from build123d import *

# Parameters (mm, degrees)
SKETCH1_W                = 50
SKETCH1_H                = 100
BOSS_EXTRUDE1_DEPTH      = 2.5
BOSS_EXTRUDE1_DEPTH_BACK = 2.5


with BuildPart() as part:
    # Sketch1 → Boss-Extrude1 (new body, two sides)
    with BuildSketch(Plane(origin=(0, 0, 0), x_dir=(1, 0, 0), z_dir=(0, 1, 0))) as boss_extrude1_sk:
        Rectangle(SKETCH1_W, SKETCH1_H)
        with BuildLine():
            Line((4.7625, 35.2375), (4.7625, -35.2375))
            ThreePointArc((4.7625, -35.2375), (0, -40), (-4.7625, -35.2375))
            Line((-4.7625, -35.2375), (-4.7625, 35.2375))
            ThreePointArc((-4.7625, 35.2375), (0, 40), (4.7625, 35.2375))
        make_face(mode=Mode.SUBTRACT)
    extrude(amount=BOSS_EXTRUDE1_DEPTH)
    extrude(boss_extrude1_sk.sketch, amount=-BOSS_EXTRUDE1_DEPTH_BACK)


solid = part.part
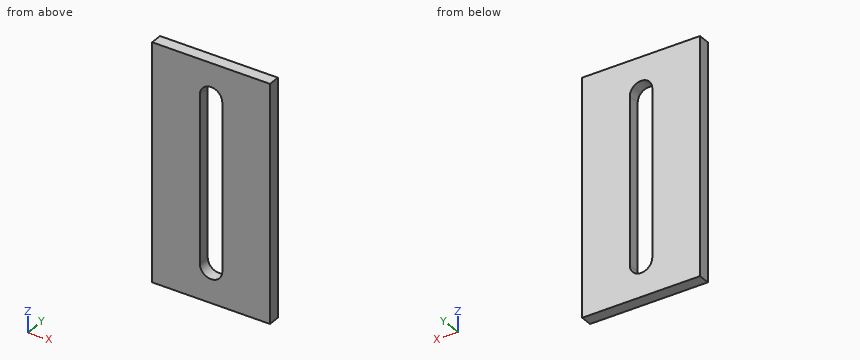
The listing builds one solid part. Answer for the finished solid, in the listing's coordinates (mm). Round coordinates to 2 decimals unless told otherwise and drop trailing zeros. Write each loop counter-clockwise with the first axis right and the second up, starting at its lowest first coordinate (ties: lowest second). Pieces come first, ordered by that corner, then holes. Notation, with made-up numbers: M -24,0 L 5,0 A14 ccw 5,27 Z; hole C -34.75,35.25 d3. An arc over 180 degrees is marked long. Write each question's results on one line, items separated by ' | '. Start each with the question number.
(1) The part is cut by section C-C, the plane z = 12.5. Write down the section's boundary in (x, y), and give its area (3 significant figures).
(2) Each of these flat-tipped pins is pushed along its axis until it touches: P1, Ø12, axis at x = 3.5, z = -4.5, coming from the +Y side; P2, Ø1, axis at x = 4, z = 36, coming from the -Y side. Where does it stop, or does it pass through?
(3) The part is cut by section A-A, the plane x = 0. Write down the section's boundary in (y, z).
(4) The part is cut by section B-B, the plane y = -1.35. Write down the section's boundary in (x, z) (1 decimal), and give its area (3 significant figures).
(5) Find the intervals of material crossed by line 1 (X direction, y = 1.9, z = 23); line 2 (X direction, y = -0.3, z = -37); line 3 (Z direction, x = 4, y = -0.5), in increasing order.
Worked answers:
1) outline: M -25,-2.5 L -4.76,-2.5 L -4.76,2.5 L -25,2.5 Z; M 4.76,-2.5 L 25,-2.5 L 25,2.5 L 4.76,2.5 Z | area: 202 mm²
2) P1: stops at y = 2.5 | P2: passes through
3) outline: M -2.5,-50 L 2.5,-50 L 2.5,-40 L -2.5,-40 Z; M -2.5,40 L 2.5,40 L 2.5,50 L -2.5,50 Z
4) outline: M -25,-50 L 25,-50 L 25,50 L -25,50 Z; hole M -4.8,-35.2 A4.8 ccw 4.8,-35.2 L 4.8,35.2 A4.8 ccw -4.8,35.2 Z | area: 4,260 mm²
5) line 1: x = -25 to -4.76, 4.76 to 25 | line 2: x = -25 to -4.42, 4.42 to 25 | line 3: z = -50 to -37.82, 37.82 to 50
